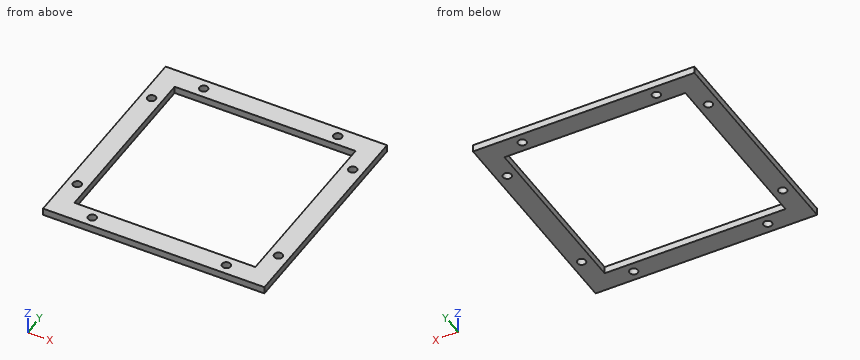
from build123d import *

# Parameters (mm, degrees)
SKETCH_W   = 93
SKETCH_H   = 93
SKETCH_R   = 1.75
SKETCH_W_2 = 76
SKETCH_H_2 = 76
PAD_DEPTH  = 3


with BuildPart() as part:
    # Sketch → Pad (new body)
    with BuildSketch(Plane.XY):
        Rectangle(SKETCH_W, SKETCH_H)
        with Locations((-28.166667, 42.25)):
            Circle(SKETCH_R, mode=Mode.SUBTRACT)
        with Locations((28.166667, 42.25)):
            Circle(SKETCH_R, mode=Mode.SUBTRACT)
        with Locations((42.25, 28.166667)):
            Circle(SKETCH_R, mode=Mode.SUBTRACT)
        with Locations((42.25, -28.166667)):
            Circle(SKETCH_R, mode=Mode.SUBTRACT)
        with Locations((28.166667, -42.25)):
            Circle(SKETCH_R, mode=Mode.SUBTRACT)
        with Locations((-28.166667, -42.25)):
            Circle(SKETCH_R, mode=Mode.SUBTRACT)
        with Locations((-42.25, -28.166667)):
            Circle(SKETCH_R, mode=Mode.SUBTRACT)
        with Locations((-42.25, 28.166667)):
            Circle(SKETCH_R, mode=Mode.SUBTRACT)
        Rectangle(SKETCH_W_2, SKETCH_H_2, mode=Mode.SUBTRACT)
    extrude(amount=PAD_DEPTH)


solid = part.part
Here's how the part is built. I have some questions about the finished solid (model axes, mm). Give positions to 0.01 mm unless a question says otherwise; leave off trailing zeros. Order: outer loops, then holes, each group sorted by start corner. A loop starts at its lowest first (then second) coordinate and runs counter-clockwise, first axis right, second up. Notation, with made-up numbers: M 37.25,34 L 94.25,34 A16 cw 94.25,65 Z; hole C 3.25,0.5 d8. An arc over 180 degrees is marked long. Answer as a JSON object with one key per item and string values. Group by question number.
1) Suppose I cut it at A-A, the plane y = 42.25. Write out the boundary of the cut face in (x, z), plus the area to 3 significant figures.
2) Please list where these lines run through material, in increasing order: L1, parallel to Y at x = -42.25, z = 0.7; L2, parallel to X at y = 42, z = 0.1; L3, parallel to X at y = 13.5, z = 1.05. Write a range as [from, to].
3) Suppose I cut it at C-C, the plane z = 2.1. Count the separate pieces of the cut face and the enclosed holes in it, plus the area to 3 significant figures.
4) I'm going to push a flat-ended pin straight in: pin 1 Ø3 at (x, y) = (28.17, -42.25) entering from -Z. Where does the tip first touch, or does it pass through?
5) Suppose I cut it at B-B, the plane x = 34. Write out the boundary of the cut face in (y, z), plus the area to 3 significant figures.
Results found:
{
 "1": {"outline": "M -46.5,0 L -29.92,0 L -29.92,3 L -46.5,3 Z; M -26.42,0 L 26.42,0 L 26.42,3 L -26.42,3 Z; M 29.92,0 L 46.5,0 L 46.5,3 L 29.92,3 Z", "area": "258 mm²"},
 "2": {"L1": "[-46.5, -29.92], [-26.42, 26.42], [29.92, 46.5]", "L2": "[-46.5, -29.9], [-26.43, 26.43], [29.9, 46.5]", "L3": "[-46.5, -38], [38, 46.5]"},
 "3": {"separate pieces": "1", "enclosed holes": "9", "area": "2,800 mm²"},
 "4": {"pin 1": "through"},
 "5": {"outline": "M -46.5,0 L -38,0 L -38,3 L -46.5,3 Z; M 38,0 L 46.5,0 L 46.5,3 L 38,3 Z", "area": "51.0 mm²"}
}
